```python
from build123d import *

# Parameters (mm, degrees)
SCHIZZO1_R        = 135
ESTRUSIONE1_DEPTH = 7
SCHIZZO2_R        = 50
SCHIZZO2_R_2      = 4
ESTRUSIONE2_DEPTH = 192.431449872


with BuildPart() as part:
    # Schizzo1 → Estrusione1 (new, symmetric)
    with BuildSketch(Plane.XY):
        Circle(SCHIZZO1_R)
    extrude(amount=ESTRUSIONE1_DEPTH, both=True)

    # Schizzo2 → Estrusione2 (cut, through all)
    with BuildSketch(Plane.XY.offset(7)):
        Circle(SCHIZZO2_R)
        with Locations((-118.84774905, 38.732577319)):
            Circle(SCHIZZO2_R_2)
        with Locations((36.145364343, 119.659987617)):
            Circle(SCHIZZO2_R_2)
        with Locations((117.072774642, -35.333125777)):
            Circle(SCHIZZO2_R_2)
        with Locations((-37.920338752, -116.260536075)):
            Circle(SCHIZZO2_R_2)
    extrude(amount=-ESTRUSIONE2_DEPTH, mode=Mode.SUBTRACT)


solid = part.part
```
The model under review builds one solid part; all positions refer to its coordinate system, in mm. Give positions to 0.01 mm unless a question says otherwise; leave off trailing zeros. Write each loop counter-clockwise with the first axis right and the second up, starting at its lowest first coordinate (ties: lowest second). Pieces come first, ordered by that corner, then holes. Notation, with made-up numbers: (39, 15.5) -> (49, 15.5) arc R19 cw to (49, 28.5) -> close; hole circle Ø11 at (60, -32). An arc over 180 degrees is marked (long way). Put each result on its own line as item: value.
(1) We need section D-D, the plane x = 87. Give the boundary of the cut face in (y, z).
Results are:
outline: (-103.23, -7) -> (103.23, -7) -> (103.23, 7) -> (-103.23, 7) -> close
(2) We need section A-A, the plane x = 0. Give the boundary of the cut face in (y, z), and give its area (3 significant figures).
Results are:
outline: (-135, -7) -> (-50, -7) -> (-50, 7) -> (-135, 7) -> close; (50, -7) -> (135, -7) -> (135, 7) -> (50, 7) -> close
area: 2,380 mm²
(3) For pin 1 Ø6 at (x, z) = (-20.5, -5) entering from +Y; pin 2 Ø2 at (x, z) = (90, -4) entering from -Y; pin 3 Ø2 at (y, z) = (-64.5, 0) entering from -X; pin 4 Ø7 at (x, y) = (117.07, -35.33) entering from -Z, all flat-tipped, find the tip position at first contact; note any pin that passes through.
Results are:
pin 1: y = 133.86
pin 2: y = -101.51
pin 3: x = -119.13
pin 4: through
(4) The part is to be moulded in two halves that separate along Y. For faces 1 (the cylindrical face through (-122.844, 38.908, 0.098)), 2 (the flat face through (-2, -58, -7)), 3 (the cylindrical face through (-107.13, -82.15, 0.1)), say which applies: pulls with the +Y half, pulls with the -Y half, needs draft (parallel to the pull), parting line crosses it, or undercut.
Results are:
face 1: undercut
face 2: needs draft
face 3: parting line crosses it
(5) We need section C-C, the plane z = 3.5. Give the boundary of the cut face in (x, y), and give its area (3 significant figures).
Results are:
outline: circle Ø270 at (0, 0); hole circle Ø8 at (-118.85, 38.73); hole circle Ø100 at (0, 0); hole circle Ø8 at (-37.92, -116.26); hole circle Ø8 at (36.15, 119.66); hole circle Ø8 at (117.07, -35.33)
area: 49,200 mm²
(6) To check wall thickness, follow probe 1 along X at (y, z) = (-1.5, -3.5); probe 2 along Y at (x, z) = (-39, 6.25); probe 3 along Y at (x, z) = (0, -0.25). State the ranges of each line that lie inside material, in increasing order. Write a range as from..to.
Results are:
probe 1: -134.99..-49.98, 49.98..134.99
probe 2: -129.24..-120.11, -112.41..-31.29, 31.29..129.24
probe 3: -135..-50, 50..135
